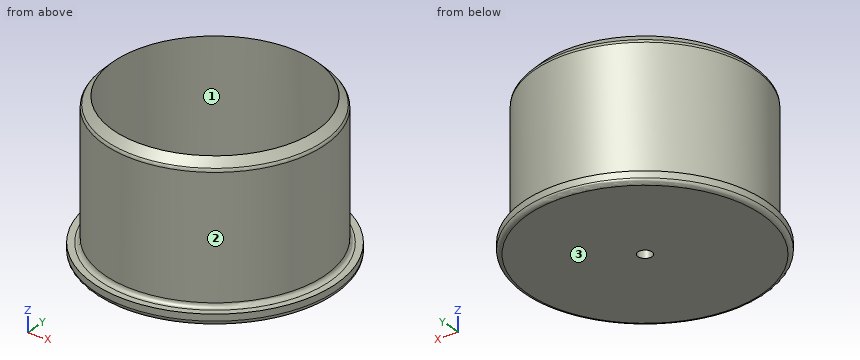
```python
from build123d import *

# Parameters (mm, degrees)
SKETCH_1_R          = 25
EXTRUDE_1_DEPTH     = 32
SKETCH_2_R          = 27.5
EXTRUDE_2_DEPTH     = 2.5
SKETCH_3_R          = 23
CUT_EXTRUDE_1_DEPTH = 32.5
CHAMFER_1_SIZE      = 3
FILLET_1_R          = 1
FILLET_2_R          = 1
FILLET_3_R          = 1
SKETCH_4_R          = 1.6
CUT_EXTRUDE_2_DEPTH = 32.5


with BuildPart() as part:
    # Эскиз1 → Бобышка-Вытянуть1 (new body)
    with BuildSketch(Plane.XY):
        Circle(SKETCH_1_R)
    extrude(amount=EXTRUDE_1_DEPTH)

    # Эскиз2 → Бобышка-Вытянуть2 (add)
    with BuildSketch(Plane(origin=(0, 0, 0), x_dir=(-1, 0, 0), z_dir=(0, 0, -1))):
        Circle(SKETCH_2_R)
    extrude(amount=EXTRUDE_2_DEPTH)

    # Эскиз3 → Вырез-Вытянуть1 (cut)
    with BuildSketch(Plane.XY.offset(32)):
        Circle(SKETCH_3_R)
    extrude(amount=-CUT_EXTRUDE_1_DEPTH, mode=Mode.SUBTRACT)

    # Фаска1
    # the kernel refuses this chamfer: 3 mm, written as the material it takes off along each edge
    with BuildSketch(Plane(origin=(0, 0, 32), x_dir=(1, 0, 0), z_dir=(0, -1, 0))) as chamfer_1_piece_1:
        Polygon((25, -CHAMFER_1_SIZE), (25 - CHAMFER_1_SIZE, 0), (25, 0), align=None)
    revolve(axis=Axis((0, 0, 32), (0, 0, 1)), mode=Mode.SUBTRACT)

    # Скругление1
    fillet_1_edges = [part.edges().sort_by_distance(p)[0] for p in [
        (-25, 0, 29),
    ]]
    fillet(fillet_1_edges, radius=FILLET_1_R)

    # Скругление2
    fillet_2_edges = [part.edges().sort_by_distance(p)[0] for p in [
        (-25, 0, 0),
    ]]
    fillet(fillet_2_edges, radius=FILLET_2_R)

    # Скругление3
    fillet_3_edges = [part.edges().sort_by_distance(p)[0] for p in [
        (27.5, 0, -2.5),
    ]]
    fillet(fillet_3_edges, radius=FILLET_3_R)

    # Эскиз4 → Вырез-Вытянуть2 (cut)
    with BuildSketch(Plane(origin=(0, 0, -2.5), x_dir=(-1, 0, 0), z_dir=(0, 0, -1))):
        Circle(SKETCH_4_R)
    extrude(amount=-CUT_EXTRUDE_2_DEPTH, mode=Mode.SUBTRACT)


solid = part.part
```
Design review of the part built by this model. Coordinates are the model's own, in mm. Face numbers are marked on the shaded views. Coordinates: 2 decimals unless noted, no trailing zeros. Order: outer loops, then holes, each group sorted by start corner. A loop starts at its lowest first (then second) coordinate and runs counter-clockwise, first axis right, second up. Notation, with made-up numbers: (8.25, 11.5) -> (21.25, 11.5) arc R24 ccw to (21.25, 27.5) -> close; hole circle Ø8 at (3, 59.5). An arc over 180 degrees is marked (long way). One line per item, written item: value. Start each with the question number.
Q1. Take a section at A-A, the plane z = 11. State the section outline as (x, y) points, then the cut area to 3 significant figures.
Q2. Insertion check: pin 1 Ø2 at (y, z) = (1, 15.5) entering from -X; pin 2 Ø1 at (y, z) = (-20, 10.5) entering from -X; pin 3 Ø5 at (y, z) = (-10.5, 25.5) entering from -X. Each pin has a flat end and moves straight along its axis. Give the tip position at first contact, or say it passes through.
Q3. For probe 1 along Y at (x, z) = (0, -1); probe 2 along Y at (x, z) = (0, 9); probe 3 along Z at (x, y) = (7.5, 20), list the stretches that pass through material, from the lowest coordinate up.
Q4. Mouldability with a two-part tool opening along X and no side actions: class the marked faces 1, 2 and 3 as pulls with the +X half, pulls with the -X half, needs draft (parallel to the pull), parting line crosses it, or undercut.
Values follow:
1. outline: circle Ø50 at (0, 0); hole circle Ø46 at (0, 0)
1. area: 302 mm2
2. pin 1: stops at x = -25
2. pin 2: stops at x = -15.64
2. pin 3: stops at x = -23.69
3. probe 1: y = -27.5 to -1.6, 1.6 to 27.5
3. probe 2: y = -25 to -23, 23 to 25
3. probe 3: z = -2.5 to -0.5
4. face 1: undercut
4. face 2: parting line crosses it
4. face 3: needs draft
